Here's how the part is built. I have some questions about the finished solid (model axes, mm). Give positions to 0.01 mm unless a question says otherwise; leave off trailing zeros. Loops run counter-clockwise (first coordinate to the right, second up) from the corner with the lowest first, then second, coordinate; pieces in that order, holes last. Notation, with made-up numbers: (6, 43.5) -> (21, 43.5) arc R20 cw to (21, 54.5) -> close; hole circle Ø6 at (46.5, 47.25). An arc over 180 degrees is marked (long way). Answer in a Markdown table with one row per item. Add a question column.
Item 1: We'd pull the mould along X, two halves only. Please class faces 1 (the face through (18.266, -90.617, 5.752)), 2 (the face through (-5.64, -89.69, 19.08)), 3 (the face through (19.5, 0, 0.5)): released by +X, released by -X, zero draft, split by the parting line, or undercut.
Item 2: If we section it at A-A (z = 5.5): Write out the boundary of the cut face in (x, y), then the cut area to 3 significant figures.
Item 3: If we section it at B-B (x = 0): Write out the boundary of the cut face in (y, z).
Item 4: If we section it at C-C (y = -26.5): Write out the boundary of the cut face in (x, z), then the cut area to 3 significant figures.
Item 5: For P1, Ø5, axis at x = -10.5, y = -117, coming from the -Z side; P2, Ø6, axis at x = 7.5, z = -13, coming from the -Y side; P3, Ø5, axis at y = -113.5, z = -9, coming from the -X side; P4, Ø1.5, axis at y = -52, z = 11.5, coming from the +X side, each with a flat end and sliding along its axis, tell me the tip position at first contact or that it passes through.
Item 6: If I drill on line 1 (Z direction, x = 0, y = -115); line 2 (X direction, y = -135.5, z = 17), over which ranges is the centre line in solid material (lowest first)?
```python
from build123d import *

# Parameters (mm, degrees)
F0_R     = 20.15
F0_R_2   = 19.15
F1_DEPTH = 150
F4_DEPTH = 151.221174
F5_DEPTH = 3.500011


with BuildPart() as f1:
    # F0 (on Front) → F1 (new body)
    with BuildSketch(Plane.XZ):
        Circle(F0_R)
        Circle(F0_R_2, mode=Mode.SUBTRACT)
    extrude(amount=F1_DEPTH)

    # F3 (on face) → F4 (cut, through all)
    with BuildSketch(Plane(origin=(0, 0, 0), x_dir=(-0.984808, 0.173648, 0), z_dir=(0.173648, 0.984808, 0))):
        with BuildLine():
            Line((0, 0), (-16.027075, -25.360064))
            ThreePointArc((-16.027075, -25.360064), (29.975998, -1.199822), (-13.948922, 26.559887))
            Line((-13.948922, 26.559887), (0, 0))
        make_face()
    extrude(amount=-F4_DEPTH, mode=Mode.SUBTRACT)

    # F3 (on face) → F5 (cut, through all)
    with BuildSketch(Plane(origin=(0, 0, 0), x_dir=(-0.984808, 0.173648, 0), z_dir=(0.173648, 0.984808, 0))):
        with BuildLine():
            Line((0, 0), (-16.027075, -25.360064))
            ThreePointArc((-16.027075, -25.360064), (29.975998, -1.199822), (-13.948922, 26.559887))
            Line((-13.948922, 26.559887), (0, 0))
        make_face()
    extrude(amount=F5_DEPTH, mode=Mode.SUBTRACT)


solid = f1.part
```
Recorded:
| question | item | result |
|---|---|---|
| 1 | face 1 | undercut |
| 1 | face 2 | released by -X |
| 1 | face 3 | zero draft |
| 2 | outline | (-19.38, -150) -> (-18.34, -150) -> (-18.34, -120.66) -> (-19.38, -126.57) -> close; (18.34, -150) -> (19.38, -150) -> (19.38, 0) -> (18.34, 0) -> close |
| 2 | area | 184 mm^2 |
| 3 | outline | (-150, -20.15) -> (-73.33, -20.15) -> (-69.7, -19.15) -> (-150, -19.15) -> close; (-150, 19.15) -> (-57.92, 19.15) -> (-60.94, 20.15) -> (-150, 20.15) -> close |
| 4 | outline | (5.16, 18.44) arc R19.15 cw to (6.81, -17.9) -> (7.36, -18.76) arc R20.15 ccw to (5.64, 19.34) -> close |
| 4 | area | 49.0 mm^2 |
| 5 | P1 | stops at z = -18.49 |
| 5 | P2 | passes through |
| 5 | P3 | stops at x = 15.31 |
| 5 | P4 | stops at x = 17.04 |
| 6 | line 1 | z = -20.15 to -19.15, 19.15 to 20.15 |
| 6 | line 2 | x = -10.82 to -8.82, 8.82 to 10.82 |
